Geometry check sheet. Reference: drawing and pictorial views, mm from the part's lowest x, y, z. Give positions to 0.01 mm unless a question says otherwise; leave off trailing zeros. Order: outer loops, then holes, each group sorted by start corner. A loop starts at its lowest first (then second) coordinate and runs counter-clockwise, first axis right, second up. Notation, with made-up numbers: (-29, -9.5) -> (25, -9.5) arc R3 cw to (25, -4.5) -> close; hole circle Ø2 at (-39, 26). An arc over 180 degrees is marked (long way). Write each question's results on one line, items separated by ' | '. Start each with the question number.
1. Mould release check, pull along Y, two halves, no side actions. Record for the marked faces 1 and 2: +Y half, -Y half, draft (parallel to the pull), parting line (faces both ways), or undercut.
2. Cross-section at B-B, the plane y = 4.5. State how many separate pieces and enclosed holes the cut face has.
3. Cross-section at C-C, the plane y = 8.5. Enter the section's corners in (x, z).
4. Material ranges on L1, parallel to X at y = 3.5, z = 0.1; L2, parallel to X at y = 3.5, z = 0.65 (1 decimal); L3, parallel to Y at x = 25, z = 0.05, recorded low to high. Write a range as from..to.
5. Cross-section at A-A, the plane z = 0.3. Enter the section's corners in (x, y), then the cut area to 3 significant figures.
6. Depth check by flat-ended pin: pin 1 Ø4.5 at (x, y) = (25, 5) entering from +Z; pin 2 Ø5 at (x, y) = (5, 5) entering from +Z. Enter the tip coordinate at first touch or a pass-through.
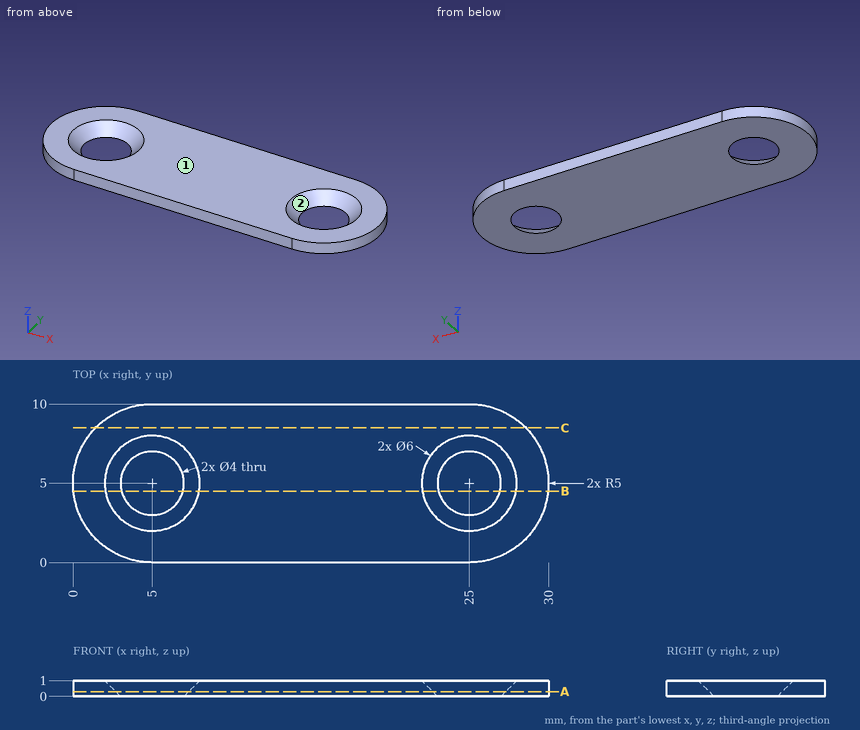
Results below:
1) face 1: draft | face 2: undercut
2) separate pieces: 3 | enclosed holes: 0
3) outline: (1.43, 0) -> (28.57, 0) -> (28.57, 1) -> (1.43, 1) -> close
4) L1: x = 0.23..3.53, 6.47..23.53, 26.47..29.77 | L2: x = 0.2..2.8, 7.2..22.8, 27.2..29.8 | L3: y = 0..2.95, 7.05..10
5) outline: (5, 0) -> (25, 0) arc R5 ccw to (25, 10) -> (5, 10) arc R5 ccw to start; hole circle Ø4.6 at (5, 5); hole circle Ø4.6 at (25, 5) | area: 245 mm²
6) pin 1: stops at z = 0.25 | pin 2: stops at z = 0.5
